The listing builds one solid part. Answer for the finished solid, in the listing's coordinates (mm). A direction names the side the tool comes from. Coordinates: 2 decimals unless noted, no trailing zeros. Order: outer loops, then holes, each group sorted by start corner. A loop starts at its lowest first (then second) coordinate and runs counter-clockwise, first axis right, second up. Notation, with made-up numbers: M 59.5,25.5 L 68.5,25.5 A6 cw 68.5,33.5 Z; hole C -29.75,-23 d1. An arc over 180 degrees is marked long. One line per item, written item: value. Start each with the question number.
Q1. Each of these flat-tipped pins is pushed along its axis until it touches: pin 1 Ø1.8 at (y, z) = (-24.5, 1.5) entering from +X; pin 2 Ø1.5 at (y, z) = (-5.5, 77.5) entering from -X; pin 3 Ø4 at (x, z) = (39.5, 33) entering from +Y. Where does it stop, or does it pass through?
Q2. For faces 4 (the flat face through (-40.524, -3, 52)), 5 (the flat face through (-25.524, -25, 20)), 6 (the cylindrical face through (-39.65, -24.4, 51.76)), 7 (the flat face through (7, -22.577, 42)), 8 (the flat face through (55, 13.423, 64)), determine the directions among +Z, -Z, +X, -X, +Y, -Y from which every point of the face is accessible in a straight line to the end or side of a thin tool.
Q3. Straight lines are drawn through the part: line 1 along X through (y, z) = (0.5, 29); line 2 along Y through (x, z) = (-35, 55.5); line 3 along X through (y, z) = (-21.5, 115). For each, find the intervals that lie inside material, in ascending order. Write a range as [from, to].
Q4. The part is cut by section B-B on y = -17. Give the vertices of the cut face in (x, z).
Q5. The part is cut by section C-C on z = 20. Give the vertices of the cut face in (x, y), then the cut area to 3 significant figures.
Q6. The part is cut by section D-D on z = 60.5. Give the vertices of the cut face in (x, y), then the cut area to 3 significant figures.
Q7. Determine the mould class of faces 1 (the cylindrical face through (54.95, -3.25, 22.48)), 2 (the cylindrical face through (-41.02, -25.15, 115.14)), 3 (the flat face through (55, -7, 5)) for opening direction Y: pulls with the +Y half, pulls with the -Y half, needs draft (parallel to the pull), parting line crosses it, or undercut.
```python
from build123d import *

# Parameters (mm, degrees)
SALIENTE_EXTRUIR1_DEPTH    = 125
CORTAR_EXTRUIR1_DEPTH      = 125
CORTAR_EXTRUIR1_DEPTH_BACK = 125
CROQUIS3_W                 = 4
CROQUIS3_H                 = 5
CROQUIS3_W_2               = 12
CROQUIS3_H_2               = 40
CROQUIS4_W                 = 91
CROQUIS4_H                 = 39
CORTAR_EXTRUIR2_DEPTH      = 125
CROQUIS5_W                 = 20
CROQUIS5_H                 = 43
SALIENTE_EXTRUIR2_DEPTH    = 2
CROQUIS6_R                 = 2.5
CORTAR_EXTRUIR3_DEPTH      = 124
CROQUIS7_R                 = 2.5
CORTAR_EXTRUIR4_DEPTH      = 124
REDONDEO1_R                = 5
REDONDEO2_R                = 5


# Some blends are built 0.0001 mm under size
with BuildPart() as part:
    # Croquis2 → Saliente-Extruir1 (new body)
    with BuildSketch(Plane.XY):
        Polygon((56.475617161, 13.42287234), (56.475617161, -26.57712766), (-40.524382839, -26.57712766), (-40.524382839, 16.42287234), (-37.524382839, 16.42287234), (-37.524382839, -22.57712766), (53.475617161, -22.57712766), (53.475617161, 13.42287234), align=None)
    extrude(amount=SALIENTE_EXTRUIR1_DEPTH)

    # Croquis3 → Cortar-Extruir1 (cut, two sides: drawn at the far end of the back side and taken through both)
    with BuildSketch(Plane(origin=(0, -22.57712766, 0), x_dir=(1, 0, 0), z_dir=(0, 1, 0)).offset(-CORTAR_EXTRUIR1_DEPTH_BACK)):
        with Locations((55.475617161, -2.5)):
            Rectangle(CROQUIS3_W, CROQUIS3_H)
        with Locations((-31.524382839, -20)):
            Rectangle(CROQUIS3_W_2, CROQUIS3_H_2)
    extrude(amount=CORTAR_EXTRUIR1_DEPTH + CORTAR_EXTRUIR1_DEPTH_BACK, mode=Mode.SUBTRACT)

    # Croquis4 → Cortar-Extruir2 (cut)
    with BuildSketch(Plane(origin=(0, -22.57712766, 0), x_dir=(1, 0, 0), z_dir=(0, 1, 0))):
        with Locations((7.975617161, -105.5)):
            Rectangle(CROQUIS4_W, CROQUIS4_H)
    extrude(amount=-CORTAR_EXTRUIR2_DEPTH, mode=Mode.SUBTRACT)

    # Croquis5 → Saliente-Extruir2 (add)
    with BuildSketch(Plane.ZY.offset(40.524382839)):
        with Locations((115, -5.07712766)):
            Rectangle(CROQUIS5_W, CROQUIS5_H)
    extrude(amount=SALIENTE_EXTRUIR2_DEPTH)

    # Croquis6 → Cortar-Extruir3 (cut)
    with BuildSketch(Plane.ZY.offset(40.524382839)):
        with Locations(Location((20, -3.57712766, 0), (0, 0, 270))):
            Circle(CROQUIS6_R)
    extrude(amount=-CORTAR_EXTRUIR3_DEPTH, mode=Mode.SUBTRACT)

    # Croquis7 → Cortar-Extruir4 (cut)
    with BuildSketch(Plane.ZY.offset(42.524382839)):
        with Locations((115, 6.42287234)):
            Circle(CROQUIS7_R)
    extrude(amount=-CORTAR_EXTRUIR4_DEPTH, mode=Mode.SUBTRACT)

    # Redondeo1
    # the kernel refuses this fillet: 5 mm, written as the material it takes off along each edge
    with BuildSketch(Plane(origin=(56.475617161, -26.57712766, -7.5), x_dir=(0, 1, 0), z_dir=(0, 0, 1))) as redondeo1_piece_1:
        with BuildLine():
            CenterArc((REDONDEO1_R, REDONDEO1_R), REDONDEO1_R, 180, 90)
            Line((0, REDONDEO1_R), (0, 0))
            Line((0, 0), (REDONDEO1_R, 0))
        make_face()
    extrude(amount=145, mode=Mode.SUBTRACT)
    with BuildSketch(Plane(origin=(-40.524382839, -26.57712766, -12.5), x_dir=(1, 0, 0), z_dir=(0, 0, 1))) as redondeo1_piece_2:
        with BuildLine():
            CenterArc((REDONDEO1_R, REDONDEO1_R), REDONDEO1_R, 180, 90)
            Line((0, REDONDEO1_R), (0, 0))
            Line((0, 0), (REDONDEO1_R, 0))
        make_face()
    extrude(amount=117.5, mode=Mode.SUBTRACT)

    # Redondeo2
    redondeo2_edges = [part.edges().sort_by_distance(p)[0] for p in [
        (-42.524382839, -26.57712766, 115),
    ]]
    fillet(redondeo2_edges, radius=REDONDEO2_R - 0.0001)  # a hair under: the kernel refuses the full size


solid = part.part
```
Output:
1. pin 1: stops at x = 53.48
1. pin 2: stops at x = -40.52
1. pin 3: stops at y = -22.58
2. face 4: -Z, -X, +Y, -Y
2. face 5: -Z, +Y, -Y
2. face 6: -Z, -X, -Y
2. face 7: +Z, -Z, +Y
2. face 8: +Z, -Z, +X, +Y
3. line 1: x = [-40.52, -37.52], [53.48, 56.48]
3. line 2: y = [-26.58, -22.58]
3. line 3: x = [-42.52, -37.52], [53.48, 56.48]
4. outline: M -42.52,105 L -40.52,105 L -40.52,0 L -37.52,0 L -37.52,125 L -42.52,125 Z; M 53.48,5 L 56.48,5 L 56.48,125 L 53.48,125 Z
5. outline: M -40.52,-21.58 A5 ccw -37.52,-26.16 L -37.52,-6.08 L -40.52,-6.08 Z; M -40.52,-1.08 L -37.52,-1.08 L -37.52,16.42 L -40.52,16.42 Z; M -25.52,-26.58 L 51.48,-26.58 A5 ccw 56.48,-21.58 L 56.48,-6.08 L 53.48,-6.08 L 53.48,-22.58 L -25.52,-22.58 Z; M 53.48,-1.08 L 56.48,-1.08 L 56.48,13.42 L 53.48,13.42 Z
5. area: 525 mm^2
6. outline: M -40.52,-21.58 A5 ccw -35.52,-26.58 L 51.48,-26.58 A5 ccw 56.48,-21.58 L 56.48,13.42 L 53.48,13.42 L 53.48,-22.58 L -37.52,-22.58 L -37.52,16.42 L -40.52,16.42 Z
6. area: 602 mm^2
7. face 1: undercut
7. face 2: pulls with the -Y half
7. face 3: needs draft
